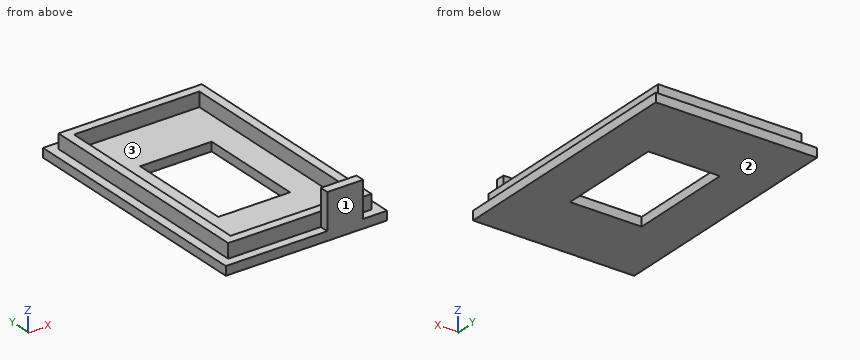
from build123d import *

# Parameters (mm, degrees)
F0_W        = 57.15
F0_H        = 88.9
F1_DEPTH    = 3.175
F2_W        = 50.8
F2_H        = 82.55
F3_DEPTH    = 5.08
F4_T        = 3.175
F4_T3_DEPTH = 57.15
F4_T5_DEPTH = 88.9
F5_W        = 25.4
F5_H        = 38.1
F6_DEPTH    = 25.4
F7_W        = 12.7
F7_H        = 7.62
F7_H_2      = 5.08
F8_DEPTH    = 3.175


# Not quite as in the source:
# - a shell that OpenCascade refuses in one call is made with other operations: the cavity is built on its own and cut out


with BuildPart() as f1:
    # F0 (on Top) → F1 (new body)
    with BuildSketch(Plane.XY):
        Rectangle(F0_W, F0_H)
    extrude(amount=F1_DEPTH)

    # F2 (on face) → F3 (join)
    with BuildSketch(Plane.XY.offset(3.175)):
        Rectangle(F2_W, F2_H)
    extrude(amount=F3_DEPTH)

    # F4: shell of thickness 3.175, made by hand


with BuildPart() as f4_core1:
    # F4_t2: copy of F1
    add(f1.part)

    # the walls: a layer under each face that stays
    f4_faces = [f4_core1.faces().sort_by_distance(p)[0] for p in [
        (0, 44.45, 1.5875),
        (28.575, 0, 1.5875),
        (-28.575, 0, 1.5875),
        (0, 0, 0),
        (-26.67, -41.4866666667, 3.175),
        (0, -44.45, 1.5875),
        (0, 41.275, 5.715),
        (-25.4, 0, 5.715),
        (0, -41.275, 5.715),
        (25.4, 0, 5.715),
    ]]
    thicken(f4_faces, amount=-F4_T, mode=Mode.SUBTRACT)

    # F4_s4 → F4_t3 (cut)
    with BuildSketch(Plane.YZ.offset(-28.575)):
        Polygon((41.30675, 3.20675), (41.275, 0), (38.1, 0), (38.1, 3.175), align=None)
        Polygon((-41.30675, 3.20675), (-41.275, 0), (-38.1, 0), (-38.1, 3.175), align=None)
    extrude(amount=F4_T3_DEPTH, mode=Mode.SUBTRACT)

    # F4_s6 → F4_t5 (cut)
    with BuildSketch(Plane.XZ.offset(-44.45)):
        Polygon((-25.43175, 3.20675), (-25.4, 0), (-22.225, 0), (-22.225, 3.175), align=None)
        Polygon((25.43175, 3.20675), (25.4, 0), (22.225, 0), (22.225, 3.175), align=None)
    extrude(amount=F4_T5_DEPTH, mode=Mode.SUBTRACT)


with BuildPart() as f1_1:
    add(f1.part)

    # what is left inside the walls is the cavity
    f4_cavity = [f4_core1.part.solids().sort_by_distance(p)[0] for p in [
        (0, -12.7, 3.20675),
    ]]
    add(f4_cavity, mode=Mode.SUBTRACT)

    # F5 (on face) → F6 (cut)
    with BuildSketch(Plane.XY.offset(3.175)):
        Rectangle(F5_W, F5_H)
    extrude(amount=-F6_DEPTH, mode=Mode.SUBTRACT)

    # F7 (on face) → F8 (join)
    with BuildSketch(Plane.XZ.offset(41.275)):
        with Locations((13.7679782532, 12.065)):
            Rectangle(F7_W, F7_H)
        with Locations((13.7679782532, 5.715)):
            Rectangle(F7_W, F7_H_2)
    extrude(amount=F8_DEPTH)


solid = f1_1.part
Input: part model. Units: mm. Frame: model coordinates. Face numbers are marked on the shaded views. Coordinates: 2 decimals unless noted, no trailing zeros. Loops run counter-clockwise (first coordinate to the right, second up) from the corner with the lowest first, then second, coordinate; pieces in that order, holes last.
Q1. Draft query along Y for the marked faces 1, 2 and 3. Return one class per face: +Y half, -Y half, draft (parallel to the pull), parting line (faces both ways), or undercut.
Q2. Contact query for flat-ended pins moving along their axis: pin 1 (4 mm diameter, centred on x = 17, y = -2.5, fed in from +Z) (3 decimals); pin 2 (5 mm diameter, centred on x = -17, z = 7, fed in from -Y) (3 decimals); pin 3 (2.5 mm diameter, centred on y = -43.5, z = 6.5, fed in from +X). Output: stop coordinate, or through.
Q3. Cut plane A-A (y = -9). Output: boundary loops of the cut face in (x, z) (3 decimals).
Q4. Material intervals for line 1 (Y direction, x = 16, z = 8) (3 decimals); line 2 (Y direction, x = 2, z = 6) (3 decimals); line 3 (X direction, y = -16.5, z = 4.75) (3 decimals), sorted ascending.
Q5. Cut plane B-B (z = 7). Output: boundary loops of the cut face in (x, y) (3 decimals), then the cut area to 3 significant figures.
Q6. Cut plane D-D (x = 18). Output: boundary loops of the cut face in (y, z) (3 decimals).
Q7. Cut plane C-C (x = -9.5). Output: boundary loops of the cut face in (y, z) (3 decimals), then the cut area to 3 significant figures.
Working result:
1. face 1: -Y half
1. face 2: draft
1. face 3: undercut
2. pin 1: stops at z = 3.175
2. pin 2: stops at y = -41.275
2. pin 3: stops at x = 20.12
3. outline: (-28.575, 0) - (-12.7, 0) - (-12.7, 3.175) - (-22.225, 3.175) - (-22.225, 8.255) - (-25.4, 8.255) - (-25.4, 3.175) - (-28.575, 3.175) - close; (12.7, 0) - (28.575, 0) - (28.575, 3.175) - (25.4, 3.175) - (25.4, 8.255) - (22.225, 8.255) - (22.225, 3.175) - (12.7, 3.175) - close
4. line 1: y = -44.45 to -38.1, 38.1 to 41.275
4. line 2: y = -41.275 to -38.1, 38.1 to 41.275
4. line 3: x = -25.4 to -22.225, 22.225 to 25.4
5. outline: (-25.4, -41.275) - (7.418, -41.275) - (7.418, -44.45) - (20.118, -44.45) - (20.118, -41.275) - (25.4, -41.275) - (25.4, 41.275) - (-25.4, 41.275) - close; hole (-22.225, -38.1) - (22.225, -38.1) - (22.225, 38.1) - (-22.225, 38.1) - close
5. area: 847 mm2
6. outline: (-44.45, 0) - (44.45, 0) - (44.45, 3.175) - (41.275, 3.175) - (41.275, 8.255) - (38.1, 8.255) - (38.1, 3.175) - (-38.1, 3.175) - (-38.1, 8.255) - (-41.275, 8.255) - (-41.275, 15.875) - (-44.45, 15.875) - close
7. outline: (-44.45, 0) - (-19.05, 0) - (-19.05, 3.175) - (-38.1, 3.175) - (-38.1, 8.255) - (-41.275, 8.255) - (-41.275, 3.175) - (-44.45, 3.175) - close; (19.05, 0) - (44.45, 0) - (44.45, 3.175) - (41.275, 3.175) - (41.275, 8.255) - (38.1, 8.255) - (38.1, 3.175) - (19.05, 3.175) - close
7. area: 194 mm2
